Work out the finished part from the listing and answer in its coordinate system (mm). Face numbers are marked on the shaded views. A direction names the side the tool comes from. Round coordinates to 2 decimals unless told otherwise and drop trailing zeros. Write each loop counter-clockwise with the first axis right and the second up, starting at its lowest first coordinate (ties: lowest second). Pieces come first, ordered by that corner, then holes. Notation, with made-up numbers: (6.5, 11.5) -> (65.5, 11.5) arc R20 ccw to (65.5, 18.5) -> close; hole circle Ø3 at (39.25, 61). An arc over 180 degrees is marked (long way). Answer as a JSON object with one key per item and string values. Group by question number.
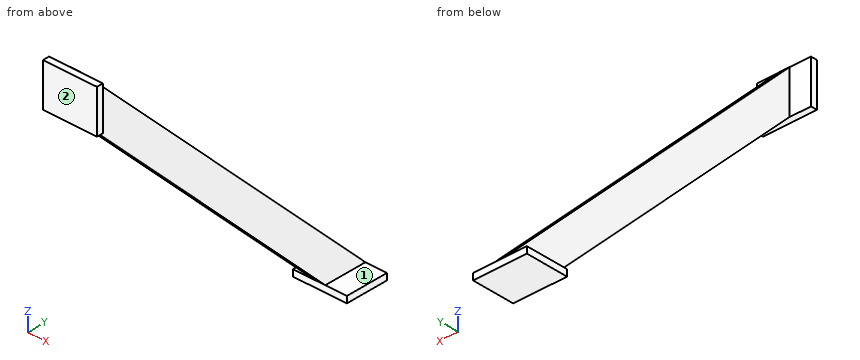
from build123d import *

# Parameters (mm, degrees)
BOSS_EXTRUDE1_DEPTH = 5
SKETCH2_W           = 25
SKETCH2_H           = 20
BOSS_EXTRUDE2_DEPTH = 3
BOSS_EXTRUDE3_DEPTH = 3


with BuildPart() as part:
    # Sketch1 → Boss-Extrude1 (new body)
    with BuildSketch(Plane(origin=(0, 0, 0), x_dir=(0, 0, -1), z_dir=(1, 0, 0))):
        Polygon((106.664666231, 114.512097991), (-34.756690006, -26.909258246), (-14.756690006, -26.909258246), (106.664666231, 94.512097991), align=None)
    extrude(amount=BOSS_EXTRUDE1_DEPTH)

    # Sketch2 → Boss-Extrude2 (add)
    with BuildSketch(Plane.XZ.offset(26.909258246)):
        with Locations((2.5, 24.703284183)):
            Rectangle(SKETCH2_W, SKETCH2_H)
    extrude(amount=BOSS_EXTRUDE2_DEPTH)

    # Sketch3 → Boss-Extrude3 (add)
    with BuildSketch(Plane(origin=(0, 0, -106.664666231), x_dir=(-1, 0, 0), z_dir=(0, 0, -1))):
        Polygon((8.72832764, 94.512097991), (10, 94.512097991), (10, 114.512097991), (-15, 114.512097991), (-15, 94.512097991), align=None)
    extrude(amount=BOSS_EXTRUDE3_DEPTH)


solid = part.part
1) A cutting plane is placed at D-D on y = 5. Determine the outline of the cut face in (x, z).
2) A cutting plane is placed at A-A on x = 9.75. Determine the outline of the cut face in (y, z).
3) Each of these flat-tipped pins is pushed along its axis until it touches: P1, Ø3.5, axis at x = -1, y = -28.5, coming from the -Z side; P2, Ø4, axis at y = 44.5, z = -53.5, coming from the -X side; P3, Ø2.5, axis at x = 8.5, z = -108.5, coming from the -Y side; P4, Ø10, axis at y = 29.5, z = -49.5, coming from the +X side. Where does it stop, or does it pass through?
4) A tool of negligible diameter and unlimited length cuts with its end or side. For the marked faces 1 and 2, from which of +Z, -Z, +X, -X, +Y, -Y can it reach the whole face along a straight path? Write none if from no direction.
5) A cutting plane is placed at B-B on y = 97.5. Determine the outline of the cut face in (x, z).
6) Straight lines are drawn through the part: L1, parallel to X at y = 101, z = -95; L2, parallel to Y at x = 0.5, z = -59; L3, parallel to Z at x = 12.25, y = 101.5. For each, find the intervals that lie inside material, in ascending order.
7) A cutting plane is placed at C-C on z = -88.5. Determine the outline of the cut face in (x, y), plus the area to 3 significant figures.
Established:
{
 "1": {"outline": "(0, -17.15) -> (5, -17.15) -> (5, 2.85) -> (0, 2.85) -> close"},
 "2": {"outline": "(-29.91, 14.7) -> (-26.91, 14.7) -> (-26.91, 34.7) -> (-29.91, 34.7) -> close; (94.51, -109.66) -> (114.51, -109.66) -> (114.51, -106.66) -> (94.51, -106.66) -> close"},
 "3": {"P1": "stops at z = 14.7", "P2": "stops at x = 0", "P3": "stops at y = 94.51", "P4": "passes through"},
 "4": {"face 1": "+Z, +X, +Y, -Y", "face 2": "+Z, -Z, +X, -X, -Y"},
 "5": {"outline": "(-10, -109.66) -> (15, -109.66) -> (15, -106.66) -> (5, -106.66) -> (5, -89.65) -> (0, -89.65) -> (0, -106.66) -> (-10, -106.66) -> close"},
 "6": {"L1": "x = 0 to 5", "L2": "y = 46.85 to 66.85", "L3": "z = -109.66 to -106.66"},
 "7": {"outline": "(0, 76.35) -> (5, 76.35) -> (5, 96.35) -> (0, 96.35) -> close", "area": "100 mm²"}
}
